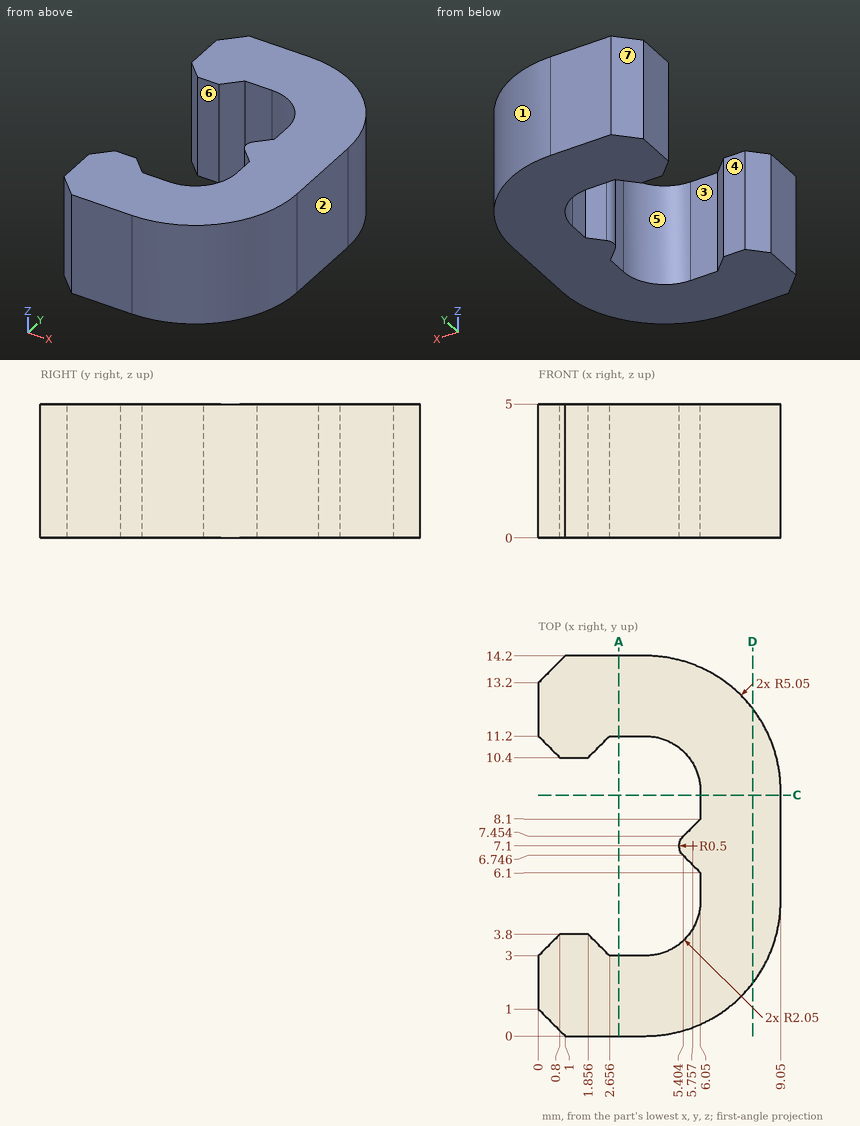
Check sheet for the drawn part. Datum: minimum x, y, z corner. Units: mm. A direction names the side the tool comes from. Coordinates: 2 decimals unless noted, no trailing zeros. Loops run counter-clockwise (first coordinate to the right, second up) from the corner with the lowest first, then second, coordinate; pieces in that order, holes last. Notation, with made-up numbers: (55.25, -17) -> (93.25, -17) arc R20 ccw to (93.25, 3) -> close; hole circle Ø5 at (55, 76.5). An arc over 180 degrees is marked (long way). Answer as CSV lines item,"result".
1) Cross-section at A-A, the plane x = 3. Record the cut outline in (y, z), then the cut area to 3 significant figures.
Found:
outline,"(0, 0) -> (3, 0) -> (3, 5) -> (0, 5) -> close; (11.2, 0) -> (14.2, 0) -> (14.2, 5) -> (11.2, 5) -> close"
area,"30.0 mm2"
2) Thickness scan on L1, parallel to X at y = 5.75, z = 4.55; L2, parallel to X at y = 10.5, z = 3.25 (1 decimal); L3, parallel to Y at x = 2.25, z = 1.8 (1 decimal). Record the ranges inside material, lowest first. Write a range as from..to.
Found:
L1,"x = 6.05..9.05"
L2,"x = 0.7..2, 5.5..8.9"
L3,"y = 0..3.4, 10.8..14.2"
3) Tool access check on the marked faces 5, 6 and 7. Record the directions out of +Z, -Z, +X, -X, +Y, -Y that give a thin tool (end or side, any length) a straight path to the whole face; none if there is none.
Found:
face 5,"+Z, -Z"
face 6,"+Z, -Z, -X"
face 7,"+Z, -Z, -X, +Y"
4) Release check for a two-part mould opening along Y. For the marked faces 1, 2, 3 and 4 record: +Y half, -Y half, draft (parallel to the pull), parting line (faces both ways), or undercut.
Found:
face 1,"+Y half"
face 2,"draft"
face 3,"undercut"
face 4,"undercut"
5) Cross-section at C-C, the plane y = 9. Record the cut outline in (x, z), then the cut area to 3 significant figures.
Found:
outline,"(6.05, 0) -> (9.05, 0) -> (9.05, 5) -> (6.05, 5) -> close"
area,"15.0 mm2"
6) Depth check by flat-ended pin: pin 1 (0.5 mm diameter, centred on y = 8.5, z = 3.5, fed in from -X). Enter the tip coordinate at first touch or a pass-through.
Found:
pin 1,"stops at x = 6.05"
7) Cross-section at D-D, the plane x = 8. Record the cut outline in (y, z).
Found:
outline,"(1.97, 0) -> (12.23, 0) -> (12.23, 5) -> (1.97, 5) -> close"
